Here's how the part is built. I have some questions about the finished solid (model axes, mm). A direction names the side the tool comes from. Coordinates: 2 decimals unless noted, no trailing zeros. Loops run counter-clockwise (first coordinate to the right, second up) from the corner with the lowest first, then second, coordinate; pieces in that order, holes last. Notation, with made-up numbers: (5.25, -37.5) -> (31.25, -37.5) arc R30 cw to (31.25, -15.5) -> close; hole circle Ø10 at (44, 35.25). An arc over 180 degrees is marked (long way). Answer as a JSON object with one key per item and string values. Group by question number.
Q1. I want a section at A-A on z = 44.45. Write out the boundary of the cut face in (x, y), then the cut area to 3 significant figures.
Q2. Thinking about a two-plate mould opening in Z: for faces 1 (the flat face through (22, -76, 88.9)), 2 (the flat face through (-92, -26, 53)), 3 (the flat face through (22, -19.65, 44)), which applies, released by +Z, released by -Z, zero draft, split by the parting line, or undercut?
Q3. I need wall thicknesses on line 1 (X direction, y = -21, z = 44); line 2 (X direction, y = -59.5, z = 44.45); line 3 (Z direction, x = 131, y = -108.5). Which ranges of each line are inside material? Lowest first, please.
Q4. I want a section at B-B on y = -44. Count the separate pieces of the cut face and the enclosed holes in it, then the cut area to 3 significant figures.
Q5. On a 3-axis mill with a long thin cutter (end or side, diameter ignored), from which of +Z, -Z, +X, -X, +Y, -Y can I reach the whole of each face in a straight line? I mean faces 4 (the flat face through (22, -133.481, 44)), 5 (the cylindrical face through (-64.89, -22.78, 41.97)). Say none if no direction works.
```python
from build123d import *

# Parameters (mm, degrees)
SKETCH1_W           = 304.8
SKETCH1_H           = 113.830905863
BOSS_EXTRUDE1_DEPTH = 88.9
SKETCH2_R           = 19.05
CUT_EXTRUDE1_DEPTH  = 6.35
SKETCH3_R           = 11.1125
CUT_EXTRUDE2_DEPTH  = 226.019242591


with BuildPart() as part:
    # Sketch1 → Boss-Extrude1 (new body)
    with BuildSketch(Plane.XY):
        with Locations((24.173793103, -76.565926378)):
            Rectangle(SKETCH1_W, SKETCH1_H)
    extrude(amount=BOSS_EXTRUDE1_DEPTH)

    # Sketch2 → Cut-Extrude1 (cut)
    with BuildSketch(Plane(origin=(0, -19.650473447, 0), x_dir=(1, 0, 0), z_dir=(0, 1, 0))):
        with Locations(Location((-83.776206897, -44.45, 0), (0, 0, 270))):
            Circle(SKETCH2_R)
        with Locations(Location((132.123793103, -44.45, 0), (0, 0, 90))):
            Circle(SKETCH2_R)
    extrude(amount=-CUT_EXTRUDE1_DEPTH, mode=Mode.SUBTRACT)

    # Sketch3 → Cut-Extrude2 (cut, through all)
    with BuildSketch(Plane(origin=(0, -26.000473447, 0), x_dir=(1, 0, 0), z_dir=(0, 1, 0))):
        with Locations(Location((-83.776206897, -44.45, 0), (0, 0, 270))):
            Circle(SKETCH3_R)
        with Locations(Location((132.123793103, -44.45, 0), (0, 0, 270))):
            Circle(SKETCH3_R)
    extrude(amount=-CUT_EXTRUDE2_DEPTH, mode=Mode.SUBTRACT)


solid = part.part
```
Result set:
{
 "1": {"outline": "(-128.23, -133.48) -> (-94.89, -133.48) -> (-94.89, -26) -> (-102.83, -26) -> (-102.83, -19.65) -> (-128.23, -19.65) -> close; (-72.66, -133.48) -> (121.01, -133.48) -> (121.01, -26) -> (113.07, -26) -> (113.07, -19.65) -> (-64.73, -19.65) -> (-64.73, -26) -> (-72.66, -26) -> close; (143.24, -133.48) -> (176.57, -133.48) -> (176.57, -19.65) -> (151.17, -19.65) -> (151.17, -26) -> (143.24, -26) -> close", "area": "29,400 mm²"},
 "2": {"face 1": "released by +Z", "face 2": "undercut", "face 3": "zero draft"},
 "3": {"line 1": "x = -128.23 to -102.82, -64.73 to 113.08, 151.17 to 176.57", "line 2": "x = -128.23 to -94.89, -72.66 to 121.01, 143.24 to 176.57", "line 3": "z = 0 to 33.39, 55.51 to 88.9"},
 "4": {"separate pieces": "1", "enclosed holes": "2", "area": "26,300 mm²"},
 "5": {"face 4": "+Z, -Z, +X, -X, -Y", "face 5": "+Y"}
}
